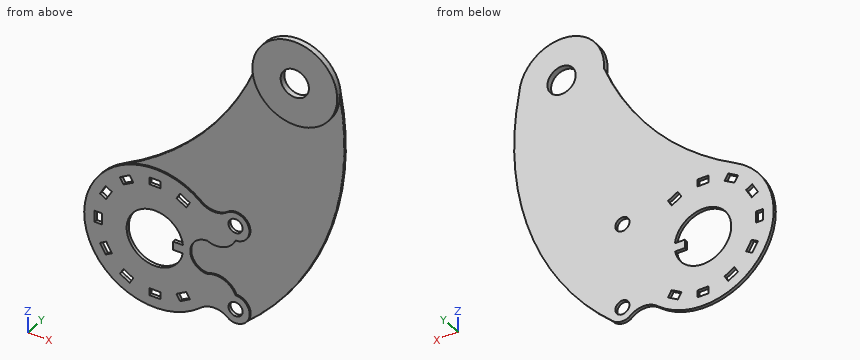
```python
from build123d import *

# Parameters (mm, degrees)
F0_R        = 5
F1_DEPTH    = 2.3
F2_DEPTH    = 1.2
F0_R_2      = 10
F3_DEPTH    = 4
F4_T4_ANGLE = 61.2690035525
F4_S5_R     = 30
F4_T6_DEPTH = 114
F4_S7_R     = 10
F4_T8_DEPTH = 114
F5_T4_ANGLE = 41.074053593
F5_S5_R     = 30
F5_T6_DEPTH = 82
F5_S7_R     = 50
F5_T8_DEPTH = 82


# Not quite as in the source:
# - a fillet or chamfer that OpenCascade refuses, or shapes differently, is made with other operations: its cross-section is extruded or revolved along the edge and cut away or added


with BuildPart() as f1:
    # F0 (on Front) → F1 (new body)
    with BuildSketch(Plane.XZ):
        with BuildLine():
            ThreePointArc((51.6923076923, 38.1603592456), (42, 34.6084670192), (32.3076923077, 38.1603592456))
            ThreePointArc((32.3076923077, 38.1603592456), (5.5214165196, 49.6942044872), (-23.1433206058, 44.3214024072))
            ThreePointArc((-23.1433206058, 44.3214024072), (-41.4946584334, -27.8961166023), (32.3076923077, -38.1603592456))
            ThreePointArc((32.3076923077, -38.1603592456), (42.5952420348, -34.6202821085), (52.5696525848, -38.9650444383))
            ThreePointArc((52.5696525848, -38.9650444383), (58.5892524469, -39.8729061912), (64.0198786028, -37.1218891035))
            ThreePointArc((64.0198786028, -37.1218891035), (66.2525372476, -26.2065115681), (57, -20))
            ThreePointArc((57, -20), (48.6934276496, -11.7664308759), (37, -12))
            ThreePointArc((37, -12), (25, 0), (37, 12))
            ThreePointArc((37, 12), (48.5892751146, 11.6008362262), (57, 19.5839644541))
            ThreePointArc((57, 19.5839644541), (66.4476997873, 32.3298447331), (51.6923076923, 38.1603592456))
        make_face()
        Polygon((-15.306354845, -34.5113842702), (-17.806354845, -38.8415112891), (-24.7345580753, -34.8415112891), (-22.1933950155, -30.4400877594), align=None, mode=Mode.SUBTRACT)
        Polygon((-30.5113842702, -22.2345580753), (-34.8415112891, -24.7345580753), (-38.8415112891, -17.806354845), (-34.4400877594, -15.2651917853), align=None, mode=Mode.SUBTRACT)
        Polygon((-37.5409129203, -4), (-42.5409129203, -4), (-42.5409129203, 4), (-37.4585868008, 4), align=None, mode=Mode.SUBTRACT)
        Polygon((3.9995764343, -37.5409085614), (3.9995764343, -42.5409129203), (-4, -42.5409129203), (-4, -37.4585868008), align=None, mode=Mode.SUBTRACT)
        Polygon((22.2341890772, -30.5115922782), (24.7341890772, -34.8417192971), (17.8063526656, -38.8415075143), (15.2651917853, -34.4400877594), align=None, mode=Mode.SUBTRACT)
        with BuildLine():
            Line((19.8513816884, 2.433648508), (12.8513816884, 2.433648508))
            Line((12.8513816884, 2.433648508), (12.8513816884, -3.566351492))
            Line((12.8513816884, -3.566351492), (19.679459775, -3.566351492))
            ThreePointArc((19.679459775, -3.566351492), (-19.9917947344, 0.572837934), (19.8513816884, 2.433648508))
        make_face(mode=Mode.SUBTRACT)
        Polygon((-34.5113842702, 15.306354845), (-38.8415112891, 17.806354845), (-34.8415112891, 24.7345580753), (-30.4400877594, 22.1933950155), align=None, mode=Mode.SUBTRACT)
        Polygon((-22.2345580753, 30.5113842702), (-24.7345580753, 34.8415112891), (-17.806354845, 38.8415112891), (-15.2651917853, 34.4400877594), align=None, mode=Mode.SUBTRACT)
        Polygon((15.306354845, 34.5113842702), (17.806354845, 38.8415112891), (24.7345580753, 34.8415112891), (22.1933950155, 30.4400877594), align=None, mode=Mode.SUBTRACT)
        Polygon((-4, 37.5409129203), (-4, 42.5409129203), (4, 42.5409129203), (4, 37.4585868008), align=None, mode=Mode.SUBTRACT)
        with Locations((57, -30)):
            Circle(F0_R, mode=Mode.SUBTRACT)
        with Locations((57, 30)):
            Circle(F0_R, mode=Mode.SUBTRACT)
    extrude(amount=F1_DEPTH)

    # F0 (on Front) → F2 (join)
    with BuildSketch(Plane.XZ):
        with BuildLine():
            ThreePointArc((-23.1433206058, 44.3214024072), (5.5214165196, 49.6942044872), (32.3076923077, 38.1603592456))
            ThreePointArc((32.3076923077, 38.1603592456), (42, 34.6084670192), (51.6923076923, 38.1603592456))
            ThreePointArc((51.6923076923, 38.1603592456), (66.4476997873, 32.3298447331), (57, 19.5839644541))
            ThreePointArc((57, 19.5839644541), (48.5892751146, 11.6008362262), (37, 12))
            ThreePointArc((37, 12), (25, 0), (37, -12))
            ThreePointArc((37, -12), (48.6934276496, -11.7664308759), (57, -20))
            ThreePointArc((57, -20), (66.2525372476, -26.2065115681), (64.0198786028, -37.1218891035))
            ThreePointArc((64.0198786028, -37.1218891035), (122.4330747785, 48.7493192224), (129.9089599648, 152.3354044245))
            ThreePointArc((129.9089599648, 152.3354044245), (129.977231351, 151.1685891188), (130, 150))
            ThreePointArc((130, 150), (101.1913208393, 120.0236634217), (70.0946163561, 147.6192377033))
            ThreePointArc((70.0946163561, 147.6192377033), (32.7491957463, 87.5998980678), (-23.1433206058, 44.3214024072))
        make_face()
    extrude(amount=F2_DEPTH)

    # F0 (on Front) → F3 (join)
    with BuildSketch(Plane.XZ):
        with BuildLine():
            ThreePointArc((129.9089599648, 152.3354044245), (97.6419159614, 179.9071804032), (70.0946163561, 147.6192377033))
            ThreePointArc((70.0946163561, 147.6192377033), (101.1913208393, 120.0236634217), (130, 150))
            ThreePointArc((130, 150), (129.977231351, 151.1685891188), (129.9089599648, 152.3354044245))
        make_face()
        with Locations((100, 150)):
            Circle(F0_R_2, mode=Mode.SUBTRACT)
    extrude(amount=F3_DEPTH)

    # F4: fillet of radius 0.25 on 1 edges, made by hand


with BuildPart() as f4_tool2:
    # F4_s3 → F4_t4 (revolve)
    with BuildSketch(Plane(origin=(17.0947609574, 0, 14.2583854823), x_dir=(0, 1, 0), z_dir=(-0.7679394892, 0, -0.6405223969))):
        with BuildLine():
            ThreePointArc((-1.2, 69.2879529885), (-1.1267766953, 69.4647296838), (-0.95, 69.5379529885))
            Line((-0.95, 69.5379529885), (-1.2, 69.5379529885))
            Line((-1.2, 69.5379529885), (-1.2, 69.2879529885))
        make_face()
    revolve(axis=Axis((-66.469102104, -1.2, 114.4453432197), (0, -1, 0)), revolution_arc=F4_T4_ANGLE)

    # F4_s5 → F4_t6 (cut, symmetric)
    with BuildSketch(Plane.XZ.offset(1)):
        with Locations((100, 150)):
            Circle(F4_S5_R)
    extrude(amount=F4_T6_DEPTH, both=True, mode=Mode.SUBTRACT)

    # F4_s7 → F4_t8 (cut, symmetric)
    with BuildSketch(Plane.XZ.offset(1)):
        with Locations((57, -30)):
            Circle(F4_S7_R)
    extrude(amount=F4_T8_DEPTH, both=True, mode=Mode.SUBTRACT)


with BuildPart() as f1_1:
    add(f1.part)

    # F4_t1: cut F4_tool2
    add(f4_tool2.part, mode=Mode.SUBTRACT)

    # F5: fillet of radius 0.25 on 1 edges, made by hand


with BuildPart() as f5_tool2:
    # F5_s3 → F5_t4 (revolve)
    with BuildSketch(Plane(origin=(60.0718928504, 0, 152.245866678), x_dir=(0, 1, 0), z_dir=(0.3670335308, 0, 0.9302077119))):
        with BuildLine():
            ThreePointArc((-1.2, -11.2723193897), (-1.1267766953, -11.0955426945), (-0.95, -11.0223193897))
            Line((-0.95, -11.0223193897), (-1.2, -11.0223193897))
            Line((-1.2, -11.0223193897), (-1.2, -11.2723193897))
        make_face()
    revolve(axis=Axis((-115.7166030288, -1.2, 221.6070120359), (0, 1, 0)), revolution_arc=F5_T4_ANGLE)

    # F5_s5 → F5_t6 (cut, symmetric)
    with BuildSketch(Plane.XZ.offset(1)):
        with Locations((100, 150)):
            Circle(F5_S5_R)
    extrude(amount=F5_T6_DEPTH, both=True, mode=Mode.SUBTRACT)

    # F5_s7 → F5_t8 (cut, symmetric)
    with BuildSketch(Plane.XZ.offset(1)):
        Circle(F5_S7_R)
    extrude(amount=F5_T8_DEPTH, both=True, mode=Mode.SUBTRACT)


with BuildPart() as f1_2:
    add(f1_1.part)

    # F5_t1: cut F5_tool2
    add(f5_tool2.part, mode=Mode.SUBTRACT)


solid = f1_2.part
```
Check sheet for the modelled part. Datum: model origin and axes. Units: mm. Round coordinates to 2 decimals unless told otherwise and drop trailing zeros. Loops run counter-clockwise (first coordinate to the right, second up) from the corner with the lowest first, then second, coordinate; pieces in that order, holes last. Notation, with made-up numbers: (83, 21.25) - (121, 21.25) arc R23 ccw to (121, 56.25) - close; hole circle Ø7 at (72, 82). An arc over 180 degrees is marked (long way). Write item = value, one per line. Start each with the question number.
Q1. Section check B-B (x = 0). Count the separate pieces of the cut face and the enclosed holes in it, plus the area to 3 significant figures.
Q2. Section check A-A (y = -3). Record the boundary of the cut face in (x, z), plus the area to 3 significant figures.
Q3. Depth check by flat-ended pin: P1, Ø1.2, axis at x = 17.5, y = -1.5, coming from the +Z side; P2, Ø10, axis at x = 112, z = 106, coming from the -Y side; P3, Ø8, axis at x = 47, z = -11.5, coming from the -Y side. Enter the tip coordinate at first touch or a pass-through.
Q4. Thickness scan on L1, parallel to Z at x = 100, y = -2.5; L2, parallel to Z at x = 99, y = -3.05; L3, parallel to Z at x = 57, y = -0.7. Record the ranges inside material, lowest first.
Derived:
q1.separate_pieces = 4
q1.enclosed_holes = 0
q1.area = 125 mm^2
q2.outline = circle Ø60 at (100, 150); hole circle Ø20 at (100, 150)
q2.area = 2,510 mm^2
q3.P1 = 72.77
q3.P2 = -1.2
q3.P3 = -2.3
q4.L1 = 120 to 140, 160 to 180
q4.L2 = 120.02 to 140.05, 159.95 to 179.98
q4.L3 = -40 to -35, -25 to 25, 35 to 120.77
